Part model, mm, in its own coordinate system. A direction names the side the tool comes from. Give positions to 0.01 mm unless a question says otherwise; leave off trailing zeros. Loops run counter-clockwise (first coordinate to the right, second up) from the corner with the lowest first, then second, coordinate; pieces in that order, holes last. Notation, with made-up numbers: (-5.75, -7.75) -> (42.25, -7.75) arc R15 cw to (42.25, 3.25) -> close; hole circle Ø4 at (14.5, 70.5). An arc over 180 degrees is marked (long way). Write item = value, one per line.
Autodesk Inventor part; units mm, degrees
ref_plane "YZ Plane" through (0, 0, 0) normal (1, 0, 0) x (0, 1, 0)
ref_plane "XZ Plane" through (0, 0, 0) normal (0, 1, 0) x (-1, 0, 0)
ref_plane "XY Plane" through (0, 0, 0) normal (0, 0, 1) x (1, 0, 0)
sketch "Sketch1" plane through (0, 0, 0) normal (1, 0, 0) x (0, 1, 0)
  line L0 (0, 0) -> (241.3, 0)
  line L1 (241.3, 0) -> (241.3, -25.4)
  line L2 (241.3, -25.4) -> (0, -25.4)
  line L3 (0, -25.4) -> (0, 0)
  line L4 (6.3489, -9.0357) -> (12.6978, -5.3677)
  line L5 (12.6978, -5.3677) -> (19.0489, -9.0319)
  line L6 (19.0489, -9.0319) -> (19.0511, -16.3643)
  line L7 (19.0511, -16.3643) -> (12.7022, -20.0323)
  line L8 (12.7022, -20.0323) -> (6.3511, -16.3681)
  line L9 (6.3511, -16.3681) -> (6.3489, -9.0357)
  point P0 (12.7, -12.7)
  dimension "d0" = 241.3
  dimension "d1" = 25.4
  dimension "d3" = 12.7
  dimension "d4" = 12.7
extrude "Extrusion1" add sketch "Sketch1" along normal blind 25.4
sketch "Sketch2" plane through (0, 241.3, 0) normal (0, 1, 0) x (1, 0, 0)
  line L0 (0, 25.4) -> (25.4, 25.4)
  line L1 (0, 0) -> (25.4, 0)
  line L2 (25.4, 0) -> (25.4, 25.4)
  line L3 (25.4, 25.4) -> (0, 25.4)
  line L4 (0, 25.4) -> (0, 0)
  line L5 (22.225, 3.175) -> (3.175, 3.175)
  line L6 (3.175, 3.175) -> (3.175, 22.225)
  line L7 (3.175, 22.225) -> (22.225, 22.225)
  line L8 (22.225, 22.225) -> (22.225, 3.175)
  dimension "d7" = 3.175
extrude "Extrusion2" cut sketch "Sketch2" against normal blind 228.6 contours L5 L6 L7 L8
sketch "Sketch3" plane through (25.4, 0, 0) normal (1, 0, 0) x (0, 0, -1)
  line L0 (0, 241.3) -> (0, 190.5)
  line L1 (0, 0) -> (0, 241.3)
  line L2 (0, 241.3) -> (-3.175, 241.3)
  line L3 (-3.175, 241.3) -> (-3.175, 190.5)
  line L4 (-3.175, 190.5) -> (0, 190.5)
  line L5 (0, 190.5) -> (0, 241.3)
  arc A0 (-3.175, 241.3) -> (-46.143, 196.9282) centre (-8.4506, 203.4185) ccw
  line L6 (-3.175, 241.3) -> (-3.175, 238.125)
  arc A1 (-3.175, 238.125) -> (-42.9327, 197.9157) centre (-7.6224, 202.7623) ccw
  line L7 (-42.9327, 197.9157) -> (-46.143, 196.9282)
  dimension "d11" = 50.8
  dimension "d13" = 3.175
  dimension "d15" = 3.175
extrude "Extrusion3" add sketch "Sketch3" against normal blind 25.4 contours L0 L4 L3 L2
sketch "Sketch4" plane through (25.4, 0, 0) normal (1, 0, 0) x (0, 0, -1)
  point P0 (0, 0)
sketch "Sketch5" plane through (25.4, 0, 0) normal (1, 0, 0) x (0, 0, -1)
  line L0 (-3.175, 241.3) -> (-3.175, 190.5)
  line L1 (-3.175, 241.3) -> (-3.175, 196.85)
  line L2 (-3.175, 196.85) -> (-41.275, 196.85)
  arc A0 (-3.175, 241.3) -> (-41.275, 196.85) centre (-8.1247, 206.989) ccw
  line L3 (-41.275, 196.85) -> (-38.5091, 198.4089)
  line L4 (-3.175, 241.3) -> (-3.175, 238.125)
  arc A1 (-3.175, 238.125) -> (-38.5091, 198.4089) centre (-8.433, 207.227) ccw
  point P0 (0, 0)
  dimension "d18" = 44.45
  dimension "d19" = 38.1
  dimension "d20" = 3.175
  dimension "d21" = 3.175
extrude "Extrusion4" add sketch "Sketch5" against normal blind 25.4 contours L0 A1 L3 A0
sketch "Sketch6" plane through (25.4, 0, 0) normal (1, 0, 0) x (0, 0, -1)
  line L0 (0, 0) -> (25.4, 0)
  line L1 (25.4, 0) -> (25.4, 241.3)
  line L2 (12.7618, 20.0321) -> (19.0807, 16.3125)
  line L3 (19.0807, 16.3125) -> (19.0189, 8.9804)
  line L4 (19.0189, 8.9804) -> (12.6382, 5.3679)
  line L5 (12.6382, 5.3679) -> (6.3193, 9.0875)
  line L6 (6.3193, 9.0875) -> (6.3811, 16.4196)
  line L7 (6.3811, 16.4196) -> (12.7618, 20.0321)
  point P0 (12.7, 12.7)
  point P1 (12.7, 12.7)
  dimension "d25" = 12.7
  dimension "d26" = 12.7
  dimension "d27" = 12.7
extrude "Extrusion5" cut sketch "Sketch6" against normal blind 25.4
sketch "Sketch7" plane through (25.4, 0, 0) normal (1, 0, 0) x (0, 0, -1)
  line L0 (0, 0) -> (0, 190.5)
  line L1 (0, 190.5) -> (-43.4485, 190.5)
  line L2 (-43.4485, 190.5) -> (-43.4485, 241.8651)
  line L3 (-43.4485, 241.8651) -> (0, 241.8651)
  line L4 (0, 241.8651) -> (0, 190.5)
extrude "Extrusion6" cut sketch "Sketch7" against normal blind 25.4
sketch "Sketch8" plane through (0, 0, -25.4) normal (0, -1, 0) x (1, 0, 0)
  line L0 (22.225, 22.225) -> (3.175, 22.225)
  line L1 (3.175, 3.175) -> (22.225, 3.175)
  line L2 (22.225, 22.225) -> (3.175, 22.225)
  line L3 (3.175, 22.225) -> (3.175, 3.175)
  line L4 (3.175, 3.175) -> (22.225, 3.175)
  line L5 (22.225, 3.175) -> (22.225, 22.225)
  point P0 (0, 25.4)
extrude "Extrusion7" cut sketch "Sketch8" against normal blind 25.4
sketch "Sketch9" plane through (25.4, 0, 0) normal (1, 0, 0) x (0, 0, -1)
  line L0 (0, 0) -> (25.4, 0)
  line L1 (9.0338, 133.35) -> (10.9985, 133.35)
  line L2 (14.4015, 133.35) -> (16.3662, 133.35)
  line L3 (12.7, 134.3323) -> (14.4015, 133.35)
  line L4 (17.3485, 131.6485) -> (19.05, 130.6662)
  line L5 (16.3662, 133.35) -> (17.3485, 131.6485)
  line L6 (19.05, 128.7015) -> (20.0323, 127)
  line L7 (19.05, 130.6662) -> (19.05, 128.7015)
  line L8 (19.05, 125.2985) -> (19.05, 123.3338)
  line L9 (20.0323, 127) -> (19.05, 125.2985)
  line L10 (17.3485, 122.3515) -> (16.3662, 120.65)
  line L11 (19.05, 123.3338) -> (17.3485, 122.3515)
  line L12 (14.4015, 120.65) -> (12.7, 119.6677)
  line L13 (16.3662, 120.65) -> (14.4015, 120.65)
  line L14 (10.9985, 120.65) -> (9.0338, 120.65)
  line L15 (12.7, 119.6677) -> (10.9985, 120.65)
  line L16 (8.0515, 122.3515) -> (6.35, 123.3338)
  line L17 (9.0338, 120.65) -> (8.0515, 122.3515)
  line L18 (6.35, 125.2985) -> (5.3677, 127)
  line L19 (6.35, 123.3338) -> (6.35, 125.2985)
  line L20 (6.35, 128.7015) -> (6.35, 130.6662)
  line L21 (5.3677, 127) -> (6.35, 128.7015)
  line L22 (8.0515, 131.6485) -> (9.0338, 133.35)
  line L23 (6.35, 130.6662) -> (8.0515, 131.6485)
  line L24 (10.9985, 133.35) -> (12.7, 134.3323)
  point P0 (12.7, 127)
  point P1 (12.7, 127)
  dimension "d35" = 127
extrude "Extrusion8" cut sketch "Sketch9" against normal blind 25.4
sketch "Sketch10" plane through (0, 0, -25.4) normal (0, 0, -1) x (-1, 0, 0)
  circle A0 centre (-12.7, 228.6) radius 3.175
  circle A1 centre (-12.7, 203.2) radius 3.175
  line L0 (0, 241.3) -> (-25.4, 241.3)
  point P0 (0, 0)
  dimension "d39" = 6.35
  dimension "d40" = 6.35
  dimension "d41" = 12.7
  dimension "d42" = 38.1
extrude "Extrusion9" cut sketch "Sketch10" against normal blind 25.4
properties part number "claw"
1) Slice it at B-B, the plane y = 99. List the corners of the cut face in (x, z) (3 decimals), and give its area (3 significant figures).
Resolved:
outline = (0, -25.4) -> (25.4, -25.4) -> (25.4, 0) -> (0, 0) -> close; hole (3.175, -22.225) -> (22.225, -22.225) -> (22.225, -3.175) -> (3.175, -3.175) -> close
area = 282 mm²
2) Which spindle directions (+Z, -Z, +X, -X, +Y, -Y) get a long thin tool onto all of the face, cutting with end or side? Do faces 1 (the face through (13, 119, -3.175)), 2 (the face through (13.11, 206.35, -1.61)). Say none if no direction does.
Resolved:
face_1 = +Y, -Y
face_2 = +Z, -Z
3) Drop a flat-ended pin along its axis: P1, Ø5, axis at x = 12.7, y = 228.6, coming from the +Z side. Give the stop position or say it passes through.
Resolved:
P1 = through
4) Drill centre lines: line 1 along Y through (x, z) = (12.7, -1.95) (3 decimals); line 2 along Z through (x, y) = (7, 122.5) (3 decimals); line 3 along X through (y, z) = (156, -5.25) (3 decimals). Where is each one in solid material? Low to high. Write a range as [from, to].
Resolved:
line_1 = [0, 200.025], [206.375, 225.425], [231.775, 241.3]
line_2 = [-25.4, -22.225], [-3.175, 0]
line_3 = [0, 3.175], [22.225, 25.4]
5) Pull direction X, two halves, no side cores. Call faces 3 (the face through (3.175, 119, -13)), 4 (the face through (0, 122, -18)), 5 (the face through (13, 122, 0)): pulls with the +X half, pulls with the -X half, needs draft (parallel to the pull), parting line crosses it, or undercut.
Resolved:
face_3 = undercut
face_4 = pulls with the -X half
face_5 = needs draft
6) Slice it at C-C, the plane y = 228.6. List the corners of the cut face in (x, z) (3 decimals), and give its area (3 significant figures).
Resolved:
outline = (0, -25.4) -> (9.525, -25.4) -> (9.525, -22.225) -> (3.175, -22.225) -> (3.175, -3.175) -> (9.525, -3.175) -> (9.525, 0) -> (0, 0) -> close; (15.875, -25.4) -> (25.4, -25.4) -> (25.4, 0) -> (15.875, 0) -> (15.875, -3.175) -> (22.225, -3.175) -> (22.225, -22.225) -> (15.875, -22.225) -> close
area = 242 mm²
7) Slice it at A-A, the plane x = 12.7. List the corners of the cut face in (y, z) (3 decimals).
Resolved:
outline = (0, -25.4) -> (200.025, -25.4) -> (200.025, -22.225) -> (0, -22.225) -> close; (0, -3.175) -> (200.025, -3.175) -> (200.025, 0) -> (0, 0) -> close; (206.375, -25.4) -> (225.425, -25.4) -> (225.425, -22.225) -> (206.375, -22.225) -> close; (206.375, -3.175) -> (225.425, -3.175) -> (225.425, 0) -> (206.375, 0) -> close; (231.775, -25.4) -> (241.3, -25.4) -> (241.3, -22.225) -> (231.775, -22.225) -> close; (231.775, -3.175) -> (241.3, -3.175) -> (241.3, 0) -> (231.775, 0) -> close
